```python
from build123d import *

# Parameters (mm, degrees)
BOSS_EXTRU_1_DEPTH      = 1.5
CONG_1_R                = 10
ESQUISSE4_R             = 8
ESQUISSE4_R_2           = 4
ESQUISSE4_R_3           = 1.5
ESQUISSE4_R_4           = 2
ENL_V_MAT_EXTRU_3_DEPTH = 3
ESQUISSE5_R             = 1.5
ENL_V_MAT_EXTRU_4_DEPTH = 230.841793557
ESQUISSE6_R             = 1.5
ENL_V_MAT_EXTRU_5_DEPTH = 230.841793557


with BuildPart() as part:
    # Esquisse1 → Boss.-Extru.1 (new body)
    with BuildSketch(Plane(origin=(0, 0, 0), x_dir=(1, 0, 0), z_dir=(0, 1, 0))):
        with BuildLine():
            Line((165, -54.556978373), (165, 55.241669751))
            Line((165, 55.241669751), (104.517749831, 160))
            Line((104.517749831, 160), (-104.517749831, 160))
            Line((-104.517749831, 160), (-165, 55.241669751))
            Line((-165, 55.241669751), (-165, -54.556978373))
            ThreePointArc((-165, -54.556978373), (-144.278322914, -96.877393783), (-112.949332972, -132.075402973))
            ThreePointArc((-112.949332972, -132.075402973), (0, -145), (112.949332972, -132.075402973))
            ThreePointArc((112.949332972, -132.075402973), (144.278322914, -96.877393783), (165, -54.556978373))
        make_face()
    extrude(amount=BOSS_EXTRU_1_DEPTH)

    # Congé1
    cong_1_edges = [part.edges().sort_by_distance(p)[0] for p in [
        (-112.949332972, 0.75, 132.075402973),
        (-165, 0.75, 54.556978373),
        (-165, 0.75, -55.241669751),
        (-104.517749831, 0.75, -160),
        (104.517749831, 0.75, -160),
        (165, 0.75, -55.241669751),
        (165, 0.75, 54.556978373),
        (112.949332972, 0.75, 132.075402973),
    ]]
    fillet(cong_1_edges, radius=CONG_1_R)

    # Esquisse4 → Enlèv. mat.-Extru.3 (cut)
    with BuildSketch(Plane(origin=(0, 1.5, 0), x_dir=(1, 0, 0), z_dir=(0, 1, 0))):
        with Locations(Location((121.838257906, 100, 0), (0, 0, 270))):
            Circle(ESQUISSE4_R)
        with Locations(Location((105.672450369, 128, 0), (0, 0, 270))):
            Circle(ESQUISSE4_R_2)
        with Locations(Location((101.922450369, 134.495190528, 0), (0, 0, 270))):
            Circle(ESQUISSE4_R_3)
        with Locations(Location((109.422450369, 121.504809472, 0), (0, 0, 270))):
            Circle(ESQUISSE4_R_3)
        with Locations(Location((-110.816043909, 103, 0), (0, 0, 270))):
            Circle(ESQUISSE4_R_3)
        with Locations(Location((95.183956091, 103, 0), (0, 0, 270))):
            Circle(ESQUISSE4_R_3)
        with Locations(Location((-27.5, 32.5, 0), (0, 0, 270))):
            Circle(ESQUISSE4_R_3)
        with Locations(Location((35, -20, 0), (0, 0, 270))):
            Circle(ESQUISSE4_R_3)
        with Locations(Location((27.5, 32.5, 0), (0, 0, 270))):
            Circle(ESQUISSE4_R_3)
        with Locations(Location((-13, -30, 0), (0, 0, 270))):
            Circle(ESQUISSE4_R_3)
        with Locations(Location((0, 0, 0), (0, 0, 270))):
            Circle(ESQUISSE4_R_4)
        with Locations(Location((-35, -20, 0), (0, 0, 270))):
            Circle(ESQUISSE4_R_3)
        with Locations(Location((13, -30, 0), (0, 0, 270))):
            Circle(ESQUISSE4_R_3)
        with Locations(Location((155, 53, 0), (0, 0, 270))):
            Circle(ESQUISSE4_R_3)
        with Locations(Location((140, -87, 0), (0, 0, 270))):
            Circle(ESQUISSE4_R_3)
        with Locations(Location((-140, -87, 0), (0, 0, 270))):
            Circle(ESQUISSE4_R_3)
        with Locations(Location((-155, 53, 0), (0, 0, 270))):
            Circle(ESQUISSE4_R_3)
        with BuildLine():
            Line((-91.816043909, 152), (76.183956091, 152))
            Line((76.183956091, 152), (76.183956091, 50))
            Line((76.183956091, 50), (5.732457975, 50))
            Line((5.732457975, 50), (2.771638598, 42.851949703))
            ThreePointArc((2.771638598, 42.851949703), (0, 41), (-2.771638598, 42.851949703))
            Line((-2.771638598, 42.851949703), (-5.732457975, 50))
            Line((-5.732457975, 50), (-91.816043909, 50))
            Line((-91.816043909, 50), (-91.816043909, 152))
        make_face()
    extrude(amount=-ENL_V_MAT_EXTRU_3_DEPTH, mode=Mode.SUBTRACT)

    # Esquisse5 → Enlèv. mat.-Extru.4 (cut, through all)
    with BuildSketch(Plane(origin=(0, 1.5, 0), x_dir=(1, 0, 0), z_dir=(0, 1, 0))):
        with Locations(Location((-30, -80, 0), (0, 0, 270))):
            Circle(ESQUISSE5_R)
        with Locations(Location((30, -80, 0), (0, 0, 90))):
            Circle(ESQUISSE5_R)
        with BuildLine():
            Line((1.5, -112), (1.5, -118))
            ThreePointArc((1.5, -118), (0, -119.5), (-1.5, -118))
            Line((-1.5, -118), (-1.5, -112))
            ThreePointArc((-1.5, -112), (0, -110.5), (1.5, -112))
        make_face()
        with BuildLine():
            Line((1.5, -127), (1.5, -133))
            ThreePointArc((1.5, -133), (0, -134.5), (-1.5, -133))
            Line((-1.5, -133), (-1.5, -127))
            ThreePointArc((-1.5, -127), (0, -125.5), (1.5, -127))
        make_face()
    extrude(amount=-ENL_V_MAT_EXTRU_4_DEPTH, mode=Mode.SUBTRACT)

    # Esquisse6 → Enlèv. mat.-Extru.5 (cut, through all)
    with BuildSketch(Plane(origin=(0, 1.5, 0), x_dir=(1, 0, 0), z_dir=(0, 1, 0))):
        with Locations(Location((-124.54257934, -80.8788967, 0), (0, 0, 270))):
            Circle(ESQUISSE6_R)
        with Locations(Location((-124.54257934, 80.8788967, 0), (0, 0, 270))):
            Circle(ESQUISSE6_R)
        with Locations(Location((124.54257934, -80.8788967, 0), (0, 0, 90))):
            Circle(ESQUISSE6_R)
        with Locations(Location((124.54257934, 80.8788967, 0), (0, 0, 90))):
            Circle(ESQUISSE6_R)
        with Locations(Location((70, -40, 0), (0, 0, 270))):
            Circle(ESQUISSE6_R)
        with Locations(Location((-70, -40, 0), (0, 0, 90))):
            Circle(ESQUISSE6_R)
    extrude(amount=-ENL_V_MAT_EXTRU_5_DEPTH, mode=Mode.SUBTRACT)


solid = part.part
```
Verification items for the finished model (mm, model axes). Coordinates: 2 decimals unless noted, no trailing zeros. Loops run counter-clockwise (first coordinate to the right, second up) from the corner with the lowest first, then second, coordinate; pieces in that order, holes last. Notation, with made-up numbers: (10, 72) - (56, 72) arc R17 cw to (56, 91) - close; hole circle Ø8 at (23.25, -38.75). An arc over 180 degrees is marked (long way). Return JSON: item names as keys, results as strings.
1. Section check A-A, the plane y = 0.4. Count the separate pieces of the cut face and the enclosed holes in it, then the cut area to 3 significant figures.
Established:
{"separate pieces": "1", "enclosed holes": "28", "area": "71,100 mm2"}
2. Mould release check, pull along X, two halves, no side actions. Record for faces 1 (the cylindrical face through (-1.56, 0.74, 144.998)), 2 (the cylindrical face through (129.77, 0.76, -101.04)), 3 (the flat face through (-135.14, 0.74, -106.96)): +X half, -X half, draft (parallel to the pull), parting line (faces both ways), or undercut.
Established:
{"face 1": "parting line", "face 2": "undercut", "face 3": "-X half"}
3. Section check B-B, the plane x = 80.5. Record the boundary of the cut face in (y, z), then the cut area to 3 significant figures.
Established:
{"outline": "(0, -160) - (1.5, -160) - (1.5, 138.48) - (0, 138.48) - close", "area": "448 mm2"}
4. Thickness scan on L1, parallel to X at y = 0.8, z = 20; L2, parallel to X at y = 0.85, z = 30; L3, parallel to X at y = 0.65, z = -53. Record the ranges inside material, lowest first.
Established:
{"L1": "x = -165 to -36.5, -33.5 to 33.5, 36.5 to 165", "L2": "x = -165 to -14.5, -11.5 to 11.5, 14.5 to 165", "L3": "x = -164.99 to -156.5, -153.5 to -91.82, 76.18 to 153.5, 156.5 to 164.99"}
